Design review of the part built by this model. Coordinates are the model's own, in mm. A direction names the side the tool comes from. Give positions to 0.01 mm unless a question says otherwise; leave off trailing zeros. Loops run counter-clockwise (first coordinate to the right, second up) from the corner with the lowest first, then second, coordinate; pieces in that order, holes last. Notation, with made-up numbers: (27.25, 49.25) - (52.25, 49.25) arc R28 cw to (52.25, 87.25) - close; hole circle Ø8 at (72.5, 7). An arc over 180 degrees is marked (long way). One line per item, written item: value. Start each with the question number.
```python
from build123d import *

# Parameters (mm, degrees)
BOSS_EXTRUDE1_DEPTH       = 19
CUT_REVOLVE_THIN4_START   = 9.090052714
CUT_REVOLVE_THIN4_DEPTH   = 0.819894572
CUT_REVOLVE_THIN4_START_2 = 9.100052714
CUT_REVOLVE_THIN4_2_DEPTH = 0.799894572
CUT_EXTRUDE1_DEPTH        = 1.5
CUT_EXTRUDE2_START        = -1.5
CUT_EXTRUDE2_DEPTH        = 1.5


with BuildPart() as part:
    # Sketch1 → Boss-Extrude1 (new body)
    with BuildSketch(Plane(origin=(0, 0, 0), x_dir=(1, 0, 0), z_dir=(0, 1, 0))):
        with BuildLine():
            Line((0, -10), (0, -11.5))
            ThreePointArc((0, -11.5), (8.131727984, -8.131727984), (11.5, 0))
            ThreePointArc((11.5, 0), (8.131727984, 8.131727984), (0, 11.5))
            Line((0, 11.5), (0, 10))
            ThreePointArc((0, 10), (7.071067812, 7.071067812), (10, 0))
            ThreePointArc((10, 0), (7.071067812, -7.071067812), (0, -10))
        make_face()
    extrude(amount=BOSS_EXTRUDE1_DEPTH)

    # Cut-Revolve-Thin4: read off the stored shape, not the designer's step
    # Cut-Revolve-Thin4 outline → Cut-Revolve-Thin4 (cut)
    with BuildSketch(Plane(origin=(0, 0, 0), x_dir=(1, 0, 0), z_dir=(0, 1, 0)).offset(CUT_REVOLVE_THIN4_START)):
        with BuildLine():
            ThreePointArc((0, -10.385), (10.385, 0), (0, 10.385))
            Line((0, 10.385), (0, 10))
            ThreePointArc((0, 10), (10, 0), (0, -10))
            Line((0, -10), (0, -10.385))
        make_face()
    extrude(amount=CUT_REVOLVE_THIN4_DEPTH, mode=Mode.SUBTRACT)

    # Sketch3 → Cut-Extrude1 (cut)
    with BuildSketch(Plane.XZ):
        with BuildLine():
            Line((0, 11.5), (0, 10))
            ThreePointArc((0, 10), (10, 0), (0, -10))
            Line((0, -10), (0, -11.5))
            ThreePointArc((0, -11.5), (11.5, 0), (0, 11.5))
        make_face()
    extrude(amount=-CUT_EXTRUDE1_DEPTH, mode=Mode.SUBTRACT)

    # Sketch4 → Cut-Extrude2 (cut)
    with BuildSketch(Plane(origin=(0, 19, 0), x_dir=(1, 0, 0), z_dir=(0, 1, 0)).offset(CUT_EXTRUDE2_START)):
        with BuildLine():
            Line((0, -10), (0, -11.5))
            ThreePointArc((0, -11.5), (11.5, 0), (0, 11.5))
            Line((0, 11.5), (0, 10))
            ThreePointArc((0, 10), (10, 0), (0, -10))
        make_face()
    extrude(amount=CUT_EXTRUDE2_DEPTH, mode=Mode.SUBTRACT)


with BuildPart() as body_2:
    # Cut-Revolve-Thin4 2 outline → Cut-Revolve-Thin4 2 (new body)
    with BuildSketch(Plane(origin=(0, 0, 0), x_dir=(1, 0, 0), z_dir=(0, 1, 0)).offset(CUT_REVOLVE_THIN4_START_2)):
        with BuildLine():
            Line((0, 10.375), (0, 10))
            ThreePointArc((0, 10), (10, 0), (0, -10))
            Line((0, -10), (0, -10.375))
            ThreePointArc((0, -10.375), (10.375, 0), (0, 10.375))
        make_face()
    extrude(amount=CUT_REVOLVE_THIN4_2_DEPTH)


solid = part.part
```
(1) Machinability: for faces 1 (the flat face through (10.2, 9.91, -0.8)), 2 (the flat face through (0, 9, 11)), which of the approach directions +Z, -Z, +X, -X, +Y, -Y give a long, thin tool a straight path to every point of the face, cutting with its end or side? Answer none if there is none.
(2) Draft analysis for pull direction Z (two halves, no side actions). For faces 3 (the flat face through (10.2, 9.09, -0.8)), 4 (the flat face through (0, 9, -11)), state which applies: pulls with the +Z half, pulls with the -Z half, needs draft (parallel to the pull), parting line crosses it, or undercut.
(3) To check wall thickness, follow L1, parallel to Y at x = 8.75, z = 5.5; L2, parallel to Z at x = 4, y = 14.75; L3, parallel to Z at x = 7.75, y = 3.25. State the ranges of each line that lie inside material, in increasing order. Write a range as from..to.
(4) Take a section at D-D on y = 8.5. State the section outline as (x, z) points, and give its area (3 significant figures).
(5) For pin 1 Ø3 at (x, y) = (4, 12.5) entering from +Z (3 decimals); pin 2 Ø1 at (x, y) = (7, 12.5) entering from -Z; pin 3 Ø1 at (y, z) = (4, -7) entering from -X, all flat-tipped, find the tip position at first contact; note any pin that passes through.
(6) Take a section at C-C on x = 6. State the section outline as (y, z) points.
(7) Take a section at B-B on z = 6.75. State the section outline as (x, y) points.
(8) Take a section at A-A on x = 1. State the section outline as (y, z) points, and give its area (3 significant figures).
Here are the results:
1. face 1: -X
1. face 2: +Z, -Z, -X, +Y, -Y
2. face 3: undercut
2. face 4: needs draft
3. L1: 1.5..9.09, 9.91..17.5
3. L2: -10.78..-9.17, 9.17..10.78
3. L3: -8.5..-6.32, 6.32..8.5
4. outline: (0, -11.5) arc R11.5 ccw to (0, 11.5) - (0, 10) arc R10 cw to (0, -10) - close
4. area: 50.7 mm²
5. pin 1: z = 11.225
5. pin 2: z = -9.49
5. pin 3: x = 6.61
6. outline: (1.5, -9.81) - (17.5, -9.81) - (17.5, -8) - (9.91, -8) - (9.91, -8.48) - (9.09, -8.48) - (9.09, -8) - (1.5, -8) - close; (1.5, 8) - (9.09, 8) - (9.09, 8.48) - (9.91, 8.48) - (9.91, 8) - (17.5, 8) - (17.5, 9.81) - (1.5, 9.81) - close
7. outline: (7.38, 1.5) - (9.31, 1.5) - (9.31, 17.5) - (7.38, 17.5) - (7.38, 9.91) - (7.89, 9.91) - (7.89, 9.09) - (7.38, 9.09) - close
8. outline: (1.5, -11.46) - (17.5, -11.46) - (17.5, -9.95) - (9.91, -9.95) - (9.91, -10.34) - (9.09, -10.34) - (9.09, -9.95) - (1.5, -9.95) - close; (1.5, 9.95) - (9.09, 9.95) - (9.09, 10.34) - (9.91, 10.34) - (9.91, 9.95) - (17.5, 9.95) - (17.5, 11.46) - (1.5, 11.46) - close
8. area: 47.6 mm²
